Source: three-view drawing plus pictorial views. Frame: mm from the lowest corner of the part. Give positions to 0.01 mm unless a question says otherwise; leave off trailing zeros. Order: outer loops, then holes, each group sorted by start corner. A loop starts at its lowest first (then second) coordinate and runs counter-clockwise, first axis right, second up. Notation, with made-up numbers: (72.5, 28.25) -> (129.5, 28.25) arc R37 ccw to (129.5, 66.25) -> close; hole circle Ø4 at (30.5, 22). An arc over 180 degrees is marked (long way). Write item = value, one per line.
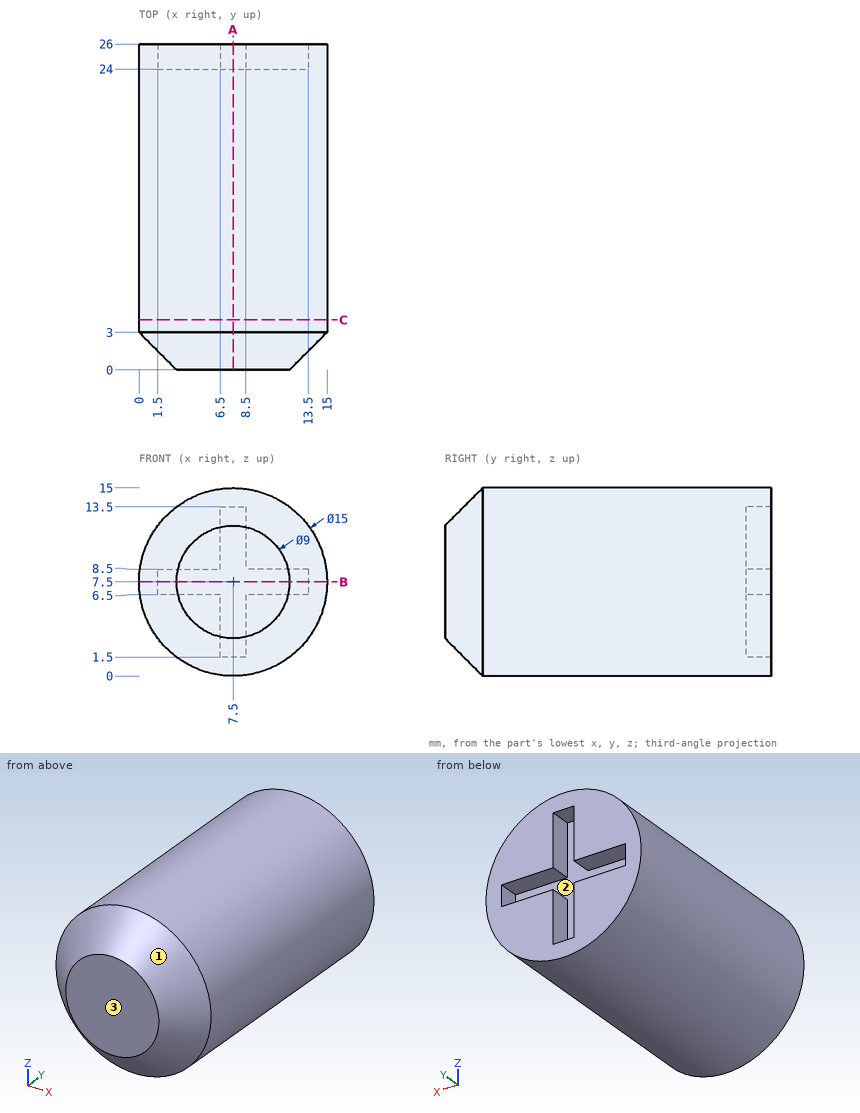
1) First-contact query: P1, Ø1, axis at y = 25, z = 5, coming from the +X side; P2, Ø2, axis at x = 4.5, y = 5, coming from the -Z side; P3, Ø1.6, axis at x = 10, y = 25.5, coming from the +Z side. Flat tips, straight axial feed; report the tip coordinate or a pass-through.
Check sheet entries:
P1 = 14.73
P2 = 0.27
P3 = 14.8
2) Line query: line 1 (Y direction, x = 4, z = 8.25); line 2 (Z direction, x = 2, y = 25.25); line 3 (X direction, y = 2.25, z = 3). Output: solid intervals per line, ascending. Write a range as from..to.
Check sheet entries:
line_1 = 0..24
line_2 = 2.4..6.5, 8.5..12.6
line_3 = 2.47..12.53
3) Section query A-A (x = 7.5). Output: boundary loops of the cut face in (y, z).
Check sheet entries:
outline = (0, 3) -> (3, 0) -> (26, 0) -> (26, 1.5) -> (24, 1.5) -> (24, 13.5) -> (26, 13.5) -> (26, 15) -> (3, 15) -> (0, 12) -> close
4) Mould query, pull axis Z, two halves, no side actions, for the marked faces 1, 2 and 3. Classes: +Z half, -Z half, draft (parallel to the pull), parting line (faces both ways), or undercut.
Check sheet entries:
face_1 = parting line
face_2 = undercut
face_3 = draft
5) Section query B-B (z = 7.5). Output: boundary loops of the cut face in (x, y).
Check sheet entries:
outline = (0, 3) -> (3, 0) -> (12, 0) -> (15, 3) -> (15, 26) -> (13.5, 26) -> (13.5, 24) -> (1.5, 24) -> (1.5, 26) -> (0, 26) -> close
6) Section query C-C (y = 4). Output: boundary loops of the cut face in (x, z).
Check sheet entries:
outline = circle Ø15 at (7.5, 7.5)
